from build123d import *

# Parameters (mm, degrees)
SKETCH1_W           = 100
SKETCH1_H           = 70
BOSS_EXTRUDE1_DEPTH = 2
SKETCH2_W           = 64
SKETCH2_H           = 49
BOSS_EXTRUDE2_DEPTH = 2
SKETCH3_R           = 2.5
CUT_EXTRUDE1_DEPTH  = 2


with BuildPart() as part:
    # Sketch1 → Boss-Extrude1 (new body)
    with BuildSketch(Plane(origin=(0, 0, 0), x_dir=(1, 0, 0), z_dir=(0, 1, 0))):
        with Locations((2.867538216, -9.96520279)):
            Rectangle(SKETCH1_W, SKETCH1_H)
    extrude(amount=BOSS_EXTRUDE1_DEPTH)

    # Sketch2 → Boss-Extrude2 (add)
    with BuildSketch(Plane(origin=(0, 2, 0), x_dir=(1, 0, 0), z_dir=(0, 1, 0))):
        with Locations((2.867538216, -9.96520279)):
            Rectangle(SKETCH2_W, SKETCH2_H)
    extrude(amount=BOSS_EXTRUDE2_DEPTH)

    # Sketch3 → Cut-Extrude1 (cut)
    with BuildSketch(Plane(origin=(0, 2, 0), x_dir=(1, 0, 0), z_dir=(0, 1, 0))):
        with Locations((-42.132461784, 7.53479721)):
            Circle(SKETCH3_R)
        with Locations((47.867538216, 7.53479721)):
            Circle(SKETCH3_R)
        with Locations((47.867538216, -27.46520279)):
            Circle(SKETCH3_R)
        with Locations((-42.132461784, -27.46520279)):
            Circle(SKETCH3_R)
    extrude(amount=-CUT_EXTRUDE1_DEPTH, mode=Mode.SUBTRACT)


solid = part.part
Here's how the part is built. I have some questions about the finished solid (model axes, mm). A direction names the side the tool comes from. Coordinates: 2 decimals unless noted, no trailing zeros. Order: outer loops, then holes, each group sorted by start corner. A loop starts at its lowest first (then second) coordinate and runs counter-clockwise, first axis right, second up. Notation, with made-up numbers: M 75,80 L 129,80 A23 cw 129,89 Z; hole C 2,-31.5 d7. An arc over 180 degrees is marked long. Answer as CSV lines item,"result". Start each with the question number.
1. For pin 1 (0.6 mm diameter, centred on x = -4, y = 3.5, fed in from -Z); pin 2 (1 mm diameter, centred on y = 3, z = 6.5, fed in from +X); pin 3 (3 mm diameter, centred on x = 47.87, z = 27.47, fed in from +Y); pin 4 (1.6 mm diameter, centred on x = -3, y = 3.5, fed in from +Z), each with a flat end and sliding along its axis, tell me the tip position at first contact or that it passes through.
2. I want a section at C-C, the plane y = 3.1. Write out the boundary of the cut face in (x, z).
3. We'd pull the mould along X, two halves only. Please class faces 1 (the flat face through (2, 3, -14.535)), 2 (the flat face through (-47.132, 1, 10)), 3 (the cylindrical face through (-42.458, 1.014, -10.014)): released by +X, released by -X, zero draft, split by the parting line, or undercut.
4. I want a section at D-D, the plane z = -20. Write out the boundary of the cut face in (x, y), and give its area (3 significant figures).
5. I need wall thicknesses on line 1 (Z direction, x = -40, y = 0.95); line 2 (Y direction, x = -34, z = 27.5); line 3 (Z direction, x = 48.5, y = 0.75). Which ranges of each line are inside material? Lowest first, please. Write a range as [from, to].
6. I want a section at B-B, the plane z = 33. Write out the boundary of the cut face in (x, y), and give its area (3 significant figures).
7. I want a section at A-A, the plane x = -8.5. Write out the boundary of the cut face in (y, z).
8. On a 3-axis mill with a long thin cutter (end or side, diameter ignored), from which of +Z, -Z, +X, -X, +Y, -Y can I reach the whole of each face in a straight line? I mean faces 4 (the cylindrical face through (46.02, 1.01, -9.22)), 5 (the flat face through (34.868, 3, 10)), 6 (the flat face through (2, 3, 34.465)), 7 (the flat face through (52.868, 1, 10)), 8 (the flat face through (-29.132, 3, 10)). Say none if no direction works.
Recorded:
1,pin 1,"stops at z = -14.53"
1,pin 2,"stops at x = 34.87"
1,pin 3,"passes through"
1,pin 4,"stops at z = 34.47"
2,outline,"M -29.13,-14.53 L 34.87,-14.53 L 34.87,34.47 L -29.13,34.47 Z"
3,face 1,"zero draft"
3,face 2,"released by -X"
3,face 3,"undercut"
4,outline,"M -47.13,0 L 52.87,0 L 52.87,2 L -47.13,2 Z"
4,area,"200 mm2"
5,line 1,"z = [-25.03, -8.84], [-6.23, 26.16], [28.77, 44.97]"
5,line 2,"y = [0, 2]"
5,line 3,"z = [-25.03, -9.95], [-5.12, 25.05], [29.88, 44.97]"
6,outline,"M -47.13,0 L 52.87,0 L 52.87,2 L 34.87,2 L 34.87,4 L -29.13,4 L -29.13,2 L -47.13,2 Z"
6,area,"328 mm2"
7,outline,"M 0,-25.03 L 2,-25.03 L 2,-14.53 L 4,-14.53 L 4,34.47 L 2,34.47 L 2,44.97 L 0,44.97 Z"
8,face 4,"+Y, -Y"
8,face 5,"+Z, -Z, +X, +Y"
8,face 6,"+Z, +X, -X, +Y"
8,face 7,"+Z, -Z, +X, +Y, -Y"
8,face 8,"+Z, -Z, -X, +Y"
